Verification items for the finished model (mm, model axes). A direction names the side the tool comes from. Coordinates: 2 decimals unless noted, no trailing zeros. Order: outer loops, then holes, each group sorted by start corner. A loop starts at its lowest first (then second) coordinate and runs counter-clockwise, first axis right, second up. Notation, with made-up numbers: M 27.25,-5 L 50.25,-5 A20 cw 50.25,15 Z; hole C 26,-9.75 d8. An arc over 180 degrees is marked long. Return JSON: item names as keys, results as strings. Group by question number.
1. Set-up check for faces 1 (the flat face through (-228.6, -258, 143)), 2 (the cylindrical face through (19.272, 37.567, 22.663)), 3 (the flat face through (-3, -355.6, 10)): record each of +Z, -Z, +X, -X, +Y, -Y from which the full face is reachable in a straight line by a thin tool's end or side.
2. Material ranges on line 1 along Y through (x, z) = (31, -53); line 2 along Y through (x, z) = (-24, 59); line 3 along X through (y, z) = (-117.5, -266.5), recorded low to high.
3. Gauge pin test, flat ends, axial feed: pin 1 (3 mm diameter, centred on y = -18, z = -129, fed in from -X); pin 2 (10 mm diameter, centred on x = 7, y = -90, fed in from -Z); pin 3 (8 mm diameter, centred on x = 194.5, z = 63.5, fed in from +Y). Record the tip position at first contact, or that the pin passes through.
4. Section check C-C, the plane z = -84.5. Record the cut outline in (x, y), plus the area to 3 significant figures.
5. Section check D-D, the plane x = 167. Record the cut outline in (y, z), plus the area to 3 significant figures.
6. Section check B-B, the plane y = -181.5. Record the cut outline in (x, z), plus the area to 3 significant figures.
7. Section check A-A, the plane x = 0. Record the cut outline in (y, z), plus the area to 3 significant figures.
```python
from build123d import *

# Parameters (mm, degrees)
F0_W     = 457.2
F0_H     = 609.6
F1_DEPTH = 355.6
F3_DEPTH = 482.6
F5_DEPTH = 25.4
F6_R     = 88.9
F7_DEPTH = 76.2


with BuildPart() as f1:
    # F0 (on Front) → F1 (new body)
    with BuildSketch(Plane.XZ):
        Rectangle(F0_W, F0_H)
    extrude(amount=F1_DEPTH)

    # F2 (on face) → F3 (join)
    with BuildSketch(Plane(origin=(-228.6, 0, 0), x_dir=(0, -1, 0), z_dir=(-1, 0, 0))):
        Polygon((373.938978, -326.002896), (0, 324.883193), (-12.612531, 315.483219), (360.396054, -333.783408), align=None)
    extrude(amount=-F3_DEPTH)

    # F4 (on face) → F5 (join)
    with BuildSketch(Plane(origin=(-228.6, 0, 0), x_dir=(0, -1, 0), z_dir=(-1, 0, 0))):
        Polygon((373.938978, -326.002896), (0, 324.883193), (-12.612531, 315.483219), (360.396054, -333.783408), align=None)
    extrude(amount=F5_DEPTH)

    # F6 (on face) → F7 (join)
    with BuildSketch(Plane(origin=(0, 0, 0), x_dir=(-1, 0, 0), z_dir=(0, 1, 0))):
        with Locations((0, 109.448686)):
            Circle(F6_R)
    extrude(amount=F7_DEPTH)


solid = f1.part
```
Answers follow:
{
 "1": {"face 1": "+Z, -X, -Y", "face 2": "+Y", "face 3": "+Z, +X, -X, -Y"},
 "2": {"line 1": "-355.6 to 0", "line 2": "-355.6 to 76.2", "line 3": "-228.6 to 228.6"},
 "3": {"pin 1": "x = -228.6", "pin 2": "z = -304.8", "pin 3": "y = 0"},
 "4": {"outline": "M -254,-235.19 L -228.6,-235.19 L -228.6,-355.6 L 228.6,-355.6 L 228.6,-235.19 L 254,-235.19 L 254,-217.18 L 228.6,-217.18 L 228.6,0 L -228.6,0 L -228.6,-217.18 L -254,-217.18 Z", "area": "163,000 mm^2"},
 "5": {"outline": "M -373.94,-326 L -360.4,-333.78 L -343.74,-304.8 L 0,-304.8 L 0,293.53 L 12.61,315.48 L 0,324.88 L -11.54,304.8 L -355.6,304.8 L -355.6,-294.08 Z", "area": "218,000 mm^2"},
 "6": {"outline": "M -254,-22.39 L -228.6,-22.39 L -228.6,-304.8 L 228.6,-304.8 L 228.6,-22.39 L 254,-22.39 L 254,8.96 L 228.6,8.96 L 228.6,304.8 L -228.6,304.8 L -228.6,8.96 L -254,8.96 Z", "area": "280,000 mm^2"},
 "7": {"outline": "M -373.94,-326 L -360.4,-333.78 L -343.74,-304.8 L 0,-304.8 L 0,20.55 L 76.2,20.55 L 76.2,198.35 L 0,198.35 L 0,293.53 L 12.61,315.48 L 0,324.88 L -11.54,304.8 L -355.6,304.8 L -355.6,-294.08 Z", "area": "231,000 mm^2"}
}
